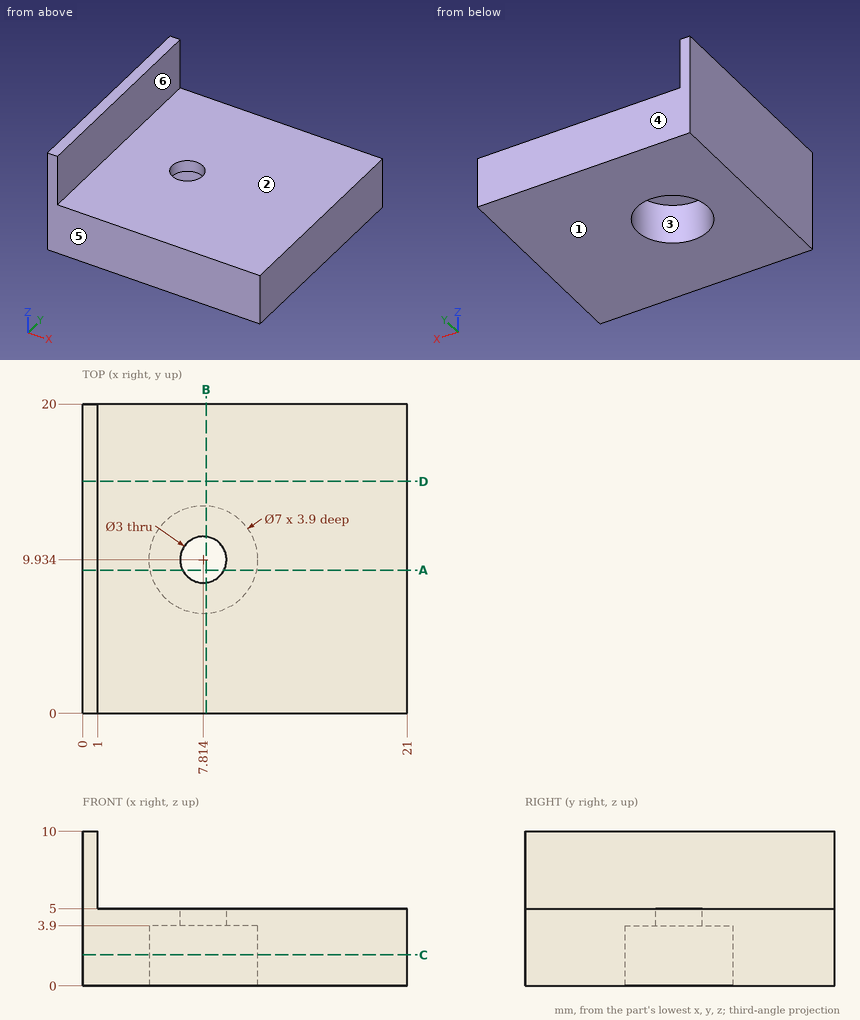
Geometry check sheet. Reference: drawing and pictorial views, mm from the part's lowest x, y, z. A direction names the side the tool comes from. Round coordinates to 2 decimals unless told otherwise and drop trailing zeros. Write each loop counter-clockwise with the first axis right and the second up, starting at its lowest first coordinate (ties: lowest second). Pieces come first, ordered by that corner, then holes.
(1) Depth check by flat-ended pin: pin 1 Ø11 at (x, y) = (7.81, 9.93) entering from +Z; pin 2 Ø2.5 at (y, z) = (13, 7.5) entering from +X; pin 3 Ø3.5 at (x, y) = (7.81, 9.93) entering from -Z. Enter the tip coordinate at first touch or a pass-through.
Returned:
pin 1: stops at z = 5
pin 2: stops at x = 1
pin 3: stops at z = 3.9
(2) Section check C-C (z = 2). Enter the section's corners in (x, y).
Returned:
outline: (0, 0) - (21, 0) - (21, 20) - (0, 20) - close; hole circle Ø7 at (7.81, 9.93)
(3) Section check B-B (x = 8). Enter the section's corners in (y, z) (1 decimal).
Returned:
outline: (0, 0) - (6.4, 0) - (6.4, 3.9) - (8.4, 3.9) - (8.4, 5) - (0, 5) - close; (11.4, 3.9) - (13.4, 3.9) - (13.4, 0) - (20, 0) - (20, 5) - (11.4, 5) - close
(4) Access from +Z, -Z, +X, -X, +Y, -Y to the whole of each face (thin tool, end or side, straight path). Record for the marked faces 1 and 2.
Returned:
face 1: -Z, +X, -X, +Y, -Y
face 2: +Z, +X, +Y, -Y
(5) Mould release check, pull along Y, two halves, no side actions. Record for the marked faces 3, 4, 5 and 6: pulls with the +Y half, pulls with the -Y half, needs draft (parallel to the pull), parting line crosses it, or undercut.
Returned:
face 3: undercut
face 4: pulls with the +Y half
face 5: pulls with the -Y half
face 6: needs draft
(6) Section check A-A (y = 9.25). Enter the section's corners in (x, z).
Returned:
outline: (0, 0) - (4.38, 0) - (4.38, 3.9) - (6.48, 3.9) - (6.48, 5) - (1, 5) - (1, 10) - (0, 10) - close; (9.15, 3.9) - (11.25, 3.9) - (11.25, 0) - (21, 0) - (21, 5) - (9.15, 5) - close
(7) Material ranges on line 1 (Z direction, x = 19.25, y = 14); line 2 (X direction, y = 9.5, z = 3.25); line 3 (X direction, y = 16.75, z = 7.75), recorded low to high.
Returned:
line 1: z = 0 to 5
line 2: x = 0 to 4.34, 11.29 to 21
line 3: x = 0 to 1
(8) Section check D-D (y = 15). Enter the section's corners in (x, z).
Returned:
outline: (0, 0) - (21, 0) - (21, 5) - (1, 5) - (1, 10) - (0, 10) - close
